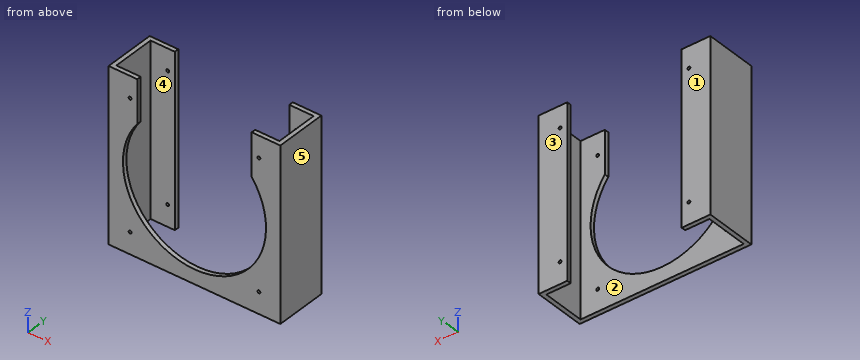
```python
from build123d import *

# Parameters (mm, degrees)
BOSS_EXTRUDE1_DEPTH      = 60
BOSS_EXTRUDE1_DEPTH_BACK = 60
SKETCH1_W                = 120
SKETCH1_H                = 36
SKETCH2_W                = 114
SKETCH2_H                = 30
CUT_EXTRUDE1_DEPTH       = 136.366170072
SKETCH3_W                = 80
SKETCH3_H                = 22.357813814
CUT_EXTRUDE2_DEPTH       = 136.366170072
SKETCH4_R                = 50
CUT_EXTRUDE3_DEPTH       = 92.043945433
SKETCH7_R                = 1
CUT_EXTRUDE4_DEPTH       = 93.173748974
CUT_EXTRUDE6_REACH       = 94.174
SKETCH9_W                = 80
SKETCH9_H                = 60


with BuildPart() as part:
    # Sketch1 → Boss-Extrude1 (new, two sides: drawn at the far end of the back side and taken through both)
    with BuildSketch(Plane.XY.offset(-BOSS_EXTRUDE1_DEPTH_BACK)):
        Rectangle(SKETCH1_W, SKETCH1_H)
    extrude(amount=BOSS_EXTRUDE1_DEPTH + BOSS_EXTRUDE1_DEPTH_BACK)

    # Sketch2 → Cut-Extrude1 (cut, through all)
    with BuildSketch(Plane.XY.offset(60)):
        Rectangle(SKETCH2_W, SKETCH2_H)
    extrude(amount=-CUT_EXTRUDE1_DEPTH, mode=Mode.SUBTRACT)

    # Sketch3 → Cut-Extrude2 (cut, through all)
    with BuildSketch(Plane.XY.offset(60)):
        with Locations((0, 15)):
            Rectangle(SKETCH3_W, SKETCH3_H)
    extrude(amount=-CUT_EXTRUDE2_DEPTH, mode=Mode.SUBTRACT)

    # Sketch4 → Cut-Extrude3 (cut, through all)
    with BuildSketch(Plane(origin=(0, -15, 0), x_dir=(1, 0, 0), z_dir=(0, 1, 0))):
        with Locations(Location((0, 0, 0), (0, 0, 270))):
            Circle(SKETCH4_R)
    extrude(amount=-CUT_EXTRUDE3_DEPTH, mode=Mode.SUBTRACT)

    # Sketch7 → Cut-Extrude4 (cut, through all)
    with BuildSketch(Plane(origin=(0, -18, 0), x_dir=(-1, 0, 0), z_dir=(0, -1, 0))):
        with Locations(Location((45, -45, 0), (0, 0, 180))):
            Circle(SKETCH7_R)
        with Locations(Location((-45, -45, 0), (0, 0, 180))):
            Circle(SKETCH7_R)
        with Locations(Location((-45, 45, 0), (0, 0, 180))):
            Circle(SKETCH7_R)
        with Locations(Location((45, 45, 0), (0, 0, 180))):
            Circle(SKETCH7_R)
    extrude(amount=-CUT_EXTRUDE4_DEPTH, mode=Mode.SUBTRACT)

    # Sketch9 → Cut-Extrude6 (cut, up to next)
    with BuildSketch(Plane.XZ.offset(18), mode=Mode.PRIVATE) as cut_extrude6_sk1:
        with Locations((0, 60)):
            Rectangle(SKETCH9_W, SKETCH9_H)
    cut_extrude6_tool1 = extrude(cut_extrude6_sk1.sketch, amount=-CUT_EXTRUDE6_REACH, mode=Mode.PRIVATE) & part.part
    add(cut_extrude6_tool1.solids().sort_by_distance((0, -18, 60))[0], mode=Mode.SUBTRACT)


solid = part.part
```
Verification items for the finished model (mm, model axes). Face numbers are marked on the shaded views. A direction names the side the tool comes from. Coordinates: 2 decimals unless noted, no trailing zeros. Write each loop counter-clockwise with the first axis right and the second up, starting at its lowest first coordinate (ties: lowest second). Pieces come first, ordered by that corner, then holes. Notation, with made-up numbers: (11, -39.5) - (23, -39.5) arc R34 cw to (23, -3.5) - close; hole circle Ø8 at (43.25, 48). An arc over 180 degrees is marked (long way). Write item = value, one per line.
Q1. Go/stop test with flat-tipped pins: pin 1 Ø10 at (x, y) = (-33, 12.5) entering from -Z; pin 2 Ø2.5 at (x, z) = (45, 45) entering from +Y. Record where each tip stops, or that it passes through.
Answer:
pin_1 = through
pin_2 = 18
Q2. Mould release check, pull along X, two halves, no side actions. Record for the marked faces 3, 4 and 5: released by +X, released by -X, zero draft, split by the parting line, or undercut.
Answer:
face_3 = zero draft
face_4 = undercut
face_5 = released by +X
Q3. Cross-section at D-D (x = 0). Enter the section's corners in (y, z).
Answer:
outline = (-18, -60) - (-15, -60) - (-15, -50) - (-18, -50) - close
Q4. Access from +Z, -Z, +X, -X, +Y, -Y to the whole of each face (thin tool, end or side, straight path). Record for the marked faces 1 and 2.
Answer:
face_1 = +Z, -Z, +X, -X, +Y
face_2 = +Z, -Z
Q5. Cross-section at B-B (z = 0). Enter the section's corners in (x, y).
Answer:
outline = (-60, -18) - (-50, -18) - (-50, -15) - (-57, -15) - (-57, 15) - (-40, 15) - (-40, 18) - (-60, 18) - close; (40, 15) - (57, 15) - (57, -15) - (50, -15) - (50, -18) - (60, -18) - (60, 18) - (40, 18) - close
Q6. Cross-section at C-C (z = 37.5). Enter the section's corners in (x, y), plus the area to 3 significant figures.
Answer:
outline = (-60, -18) - (-40, -18) - (-40, -15) - (-57, -15) - (-57, 15) - (-40, 15) - (-40, 18) - (-60, 18) - close; (40, -18) - (60, -18) - (60, 18) - (40, 18) - (40, 15) - (57, 15) - (57, -15) - (40, -15) - close
area = 420 mm²
Q7. Material ranges on L1, parallel to Z at x = 45, y = 16; L2, parallel to X at y = 1, z = 33; L3, parallel to Y at x = -50.5, z = 5.5, recorded low to high. Write a range as from..to.
Answer:
L1 = -60..-46, -44..44, 46..60
L2 = -60..-57, 57..60
L3 = -18..-15, 15..18
Q8. Cross-section at A-A (y = 4.5). Enter the section's corners in (x, z), plus the area to 3 significant figures.
Answer:
outline = (-60, -60) - (-57, -60) - (-57, 60) - (-60, 60) - close; (57, -60) - (60, -60) - (60, 60) - (57, 60) - close
area = 720 mm²
